Source: CAD feature listing. Evaluate the final solid. Frame: model axes, mm. Face numbers are marked on the shaded views. Round coordinates to 2 decimals unless told otherwise and drop trailing zeros. Loops run counter-clockwise (first coordinate to the right, second up) from the corner with the lowest first, then second, coordinate; pieces in that order, holes last.
(1) First-contact query: pin 1 Ø2.5 at (x, y) = (-7.5, 7.55) entering from +Z. Flat tip, straight axial feed; report the tip coordinate or a pass-through.
(2) Section C-C, the plane z = 1.4. Return the cut outline in (x, y).
(3) Material intervals for probe 1 along X at (y, z) = (7.75, 3.3); probe 2 along Y at (x, z) = (7.5, 2); probe 3 along X at (y, z) = (8.25, 2.4), sorted ascending.
(4) Section A-A, the plane x = 7.5. Return the cut outline in (y, z), plus the area to 3 significant figures.
(5) Section B-B, the plane y = 7.55. Return the cut outline in (x, z).
(6) Mould query, pull axis X, two halves, no side actions, for the marked faces 1, 2, 3 and 4. Classes: pulls with the +X half, pulls with the -X half, needs draft (parallel to the pull), parting line crosses it, or undercut.
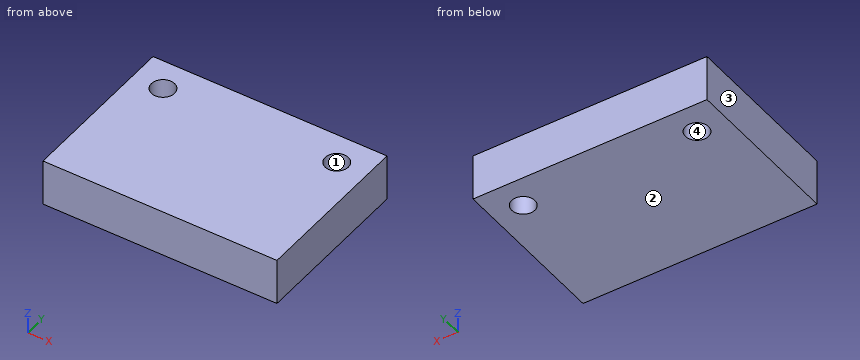
```python
from build123d import *

# Parameters (mm, degrees)
SKETCH1_W           = 20.2
SKETCH1_H           = 20.2
SKETCH1_R           = 1
BOSS_EXTRUDE1_DEPTH = 4
SKETCH2_R           = 7
SKETCH2_R_2         = 4
CUT_EXTRUDE1_DEPTH  = 4
SKETCH3_R           = 4
BOSS_EXTRUDE2_DEPTH = 4
SKETCH4_W           = 20.2
SKETCH4_H           = 6
CUT_EXTRUDE2_DEPTH  = 10


with BuildPart() as part:
    # Sketch1 → Boss-Extrude1 (new body)
    with BuildSketch(Plane.XY):
        with Locations((0, 0.05)):
            Rectangle(SKETCH1_W, SKETCH1_H)
        with Locations((7.5, 7.55)):
            Circle(SKETCH1_R, mode=Mode.SUBTRACT)
        with Locations(Location((-7.5, 7.55, 0), (0, 0, 180))):
            Circle(SKETCH1_R, mode=Mode.SUBTRACT)
        with Locations((7.5, -8.7)):
            Circle(SKETCH1_R, mode=Mode.SUBTRACT)
        with Locations(Location((-7.5, -8.7, 0), (0, 0, 180))):
            Circle(SKETCH1_R, mode=Mode.SUBTRACT)
    extrude(amount=BOSS_EXTRUDE1_DEPTH)

    # Sketch2 → Cut-Extrude1 (cut)
    with BuildSketch(Plane.XY.offset(4)):
        with Locations((0, -13.32)):
            Circle(SKETCH2_R)
        Circle(SKETCH2_R_2)
    extrude(amount=-CUT_EXTRUDE1_DEPTH, mode=Mode.SUBTRACT)

    # Sketch3 → Boss-Extrude2 (add)
    with BuildSketch(Plane.XY.offset(4)):
        Circle(SKETCH3_R)
    extrude(amount=-BOSS_EXTRUDE2_DEPTH)

    # Sketch4 → Cut-Extrude2 (cut)
    with BuildSketch(Plane.XY.offset(4)):
        with Locations((0, -7.05)):
            Rectangle(SKETCH4_W, SKETCH4_H)
    extrude(amount=-CUT_EXTRUDE2_DEPTH, mode=Mode.SUBTRACT)


solid = part.part
```
Output values:
1. pin 1: stops at z = 4
2. outline: (-10.1, -4.05) - (10.1, -4.05) - (10.1, 10.15) - (-10.1, 10.15) - close; hole circle Ø2 at (-7.5, 7.55); hole circle Ø2 at (7.5, 7.55)
3. probe 1: x = -10.1 to -8.48, -6.52 to 6.52, 8.48 to 10.1
3. probe 2: y = -4.05 to 6.55, 8.55 to 10.15
3. probe 3: x = -10.1 to -8.21, -6.79 to 6.79, 8.21 to 10.1
4. outline: (-4.05, 0) - (6.55, 0) - (6.55, 4) - (-4.05, 4) - close; (8.55, 0) - (10.15, 0) - (10.15, 4) - (8.55, 4) - close
4. area: 48.8 mm2
5. outline: (-10.1, 0) - (-8.5, 0) - (-8.5, 4) - (-10.1, 4) - close; (-6.5, 0) - (6.5, 0) - (6.5, 4) - (-6.5, 4) - close; (8.5, 0) - (10.1, 0) - (10.1, 4) - (8.5, 4) - close
6. face 1: undercut
6. face 2: needs draft
6. face 3: pulls with the -X half
6. face 4: undercut
